Design review of the part built by this model. Coordinates are the model's own, in mm. A direction names the side the tool comes from. Give positions to 0.01 mm unless a question says otherwise; leave off trailing zeros. Order: outer loops, then holes, each group sorted by start corner. A loop starts at its lowest first (then second) coordinate and runs counter-clockwise, first axis right, second up. Notation, with made-up numbers: M 12.5,10.25 L 61.5,10.25 A30 ccw 61.5,42.25 Z; hole C 64,32 d7. An arc over 180 degrees is marked long. Answer as a JSON object with one key per item and string values.
from build123d import *

# Parameters (mm, degrees)
F1_DEPTH = 3.175


# Not quite as in the source:
# - ends of sketch curves that miss each other by under 0.0002 mm in the source are joined


with BuildPart() as f1:
    # F0 (on Right) → F1 (new body, symmetric)
    with BuildSketch(Plane.YZ):
        with BuildLine():
            Line((3.175, -63.5), (23.8125, -63.5))
            Line((23.8125, -63.5), (23.8125, -50.8))
            Line((23.8125, -50.8), (23.8125, 57.15))
            ThreePointArc((23.8125, 57.15), (21.9533763667, 61.6393796296), (17.4646167058, 63.4999996472))
            Line((17.4646167058, 63.4999996472), (17.4625, 63.5))
            Line((17.4625, 63.5), (11.1139111112, 63.5))
            Line((11.1139111112, 63.5), (11.124494366, 158.7492930333))
            ThreePointArc((11.124494366, 158.7492930333), (9.2648719104, 163.2398771909), (4.7744944052, 165.0999985889))
            Line((4.7744944052, 165.0999985889), (-4.7498, 165.0999985889))
            ThreePointArc((-4.7498, 165.0999985889), (-9.2399280605, 163.2401266494), (-11.0998, 158.7499985889))
            Line((-11.0998, 158.7499985889), (-11.0998, 63.5))
            Line((-11.0998, 63.5), (-17.4498, 63.5))
            Line((-17.4498, 63.5), (-17.4625, 63.5))
            ThreePointArc((-17.4625, 63.5), (-21.9526280605, 61.6401280605), (-23.8125, 57.15))
            Line((-23.8125, 57.15), (-23.8125, -50.818807292))
            Line((-23.8125, -50.818807292), (-23.8125, -63.5))
            Line((-23.8125, -63.5), (-3.175, -63.5))
            Line((-3.175, -63.5), (-3.175, 63.5))
            Line((-3.175, 63.5), (3.175, 63.5))
            Line((3.175, 63.5), (3.175, -63.5))
        make_face()
        Polygon((23.8125, -50.8), (23.8125, -63.5), (31.115, -63.5), (31.115, -88.9), (50.165, -88.9), (50.165, -50.8), align=None)
        Polygon((-36.5125, -63.518807292), (-23.8125, -63.5), (-23.8125, -50.818807292), (-36.5125, -50.818807292), align=None)
    extrude(amount=F1_DEPTH, both=True)


solid = f1.part
(1) Tool access review of faces 4 (the flat face through (0, 17, -63.5)), 5 (the flat face through (0, 0, 63.5)), 6 (the flat face through (0, -30, -50.819)), 7 (the flat face through (0, 23.812, 2)): name each direction out of +Z, -Z, +X, -X, +Y, -Y from which nothing blocks a thin tool from reaching the whole face with its end or side.
Checked values:
{"face 4": "-Z, +X, -X, -Y", "face 5": "-Z, +X, -X", "face 6": "+Z, +X, -X, -Y", "face 7": "+Z, +X, -X, +Y"}
(2) We need section C-C (y = 37). Write out the cut boundary in (x, z) (3 decimals).
Checked values:
{"outline": "M -3.175,-88.9 L 3.175,-88.9 L 3.175,-50.8 L -3.175,-50.8 Z"}
(3) We need section D-D (z = 126). Write out the cut boundary in (x, y) (3 decimals), plus the area to 3 significant figures.
Checked values:
{"outline": "M -3.175,-11.1 L 3.175,-11.1 L 3.175,11.121 L -3.175,11.121 Z", "area": "141 mm^2"}
(4) We need section A-A (z = 21). Write out the cut boundary in (x, y) (1 decimal), plus the area to 3 significant figures.
Checked values:
{"outline": "M -3.2,-23.8 L 3.2,-23.8 L 3.2,-3.2 L -3.2,-3.2 Z; M -3.2,3.2 L 3.2,3.2 L 3.2,23.8 L -3.2,23.8 Z", "area": "262 mm^2"}
(5) To check wall thickness, follow L1, parallel to Y at x = -2, z = 39 (1 decimal); L2, parallel to Y at x = 1.25, z = -55 (1 decimal); L3, parallel to Y at x = 1.25, z = -64 (3 decimals). State the ranges of each line that lie inside material, in increasing order. Write a range as from..to.
Checked values:
{"L1": "y = -23.8..-3.2, 3.2..23.8", "L2": "y = -36.5..-3.2, 3.2..50.2", "L3": "y = 31.115..50.165"}
(6) Insertion check: pin 1 (1.9 mm diameter, centred on x = -0.5, z = 26.5, fed in from -Y); pin 2 (3 mm diameter, centred on x = -1, z = 10, fed in from +Y); pin 3 (8 mm diameter, centred on y = 21, z = 64.5, fed in from +X) (3 decimals); pin 4 (2 mm diameter, centred on x = 1.5, z = 138.5, fed in from -Y). Each pin has a flat end and moves straight along its axis. Give the tip position at first contact, or say it passes through.
Checked values:
{"pin 1": "stops at y = -23.81", "pin 2": "stops at y = 23.81", "pin 3": "stops at x = 3.175", "pin 4": "stops at y = -11.1"}
(7) Draft analysis for pull direction Y (two halves, no side actions). For faces 1 (the flat face through (0, -3.175, -1)), 2 (the flat face through (-3.175, -3.4, 11.7)), 3 (the cylindrical face through (0.044, 9.314, 163.19)), state which applies: +Y half, -Y half, draft (parallel to the pull), parting line (faces both ways), or undercut.
Checked values:
{"face 1": "undercut", "face 2": "draft", "face 3": "+Y half"}
